CAD build for the part. Positions are in the model's coordinates, mm. Give positions to 0.01 mm unless a question says otherwise; leave off trailing zeros. Write each loop counter-clockwise with the first axis right and the second up, starting at its lowest first coordinate (ties: lowest second). Pieces come first, ordered by that corner, then holes. Notation, with made-up numbers: (-26.5, 51.5) - (-8.5, 51.5) arc R10 cw to (-8.5, 55.5) - close; hole circle Ø8 at (43, -17.5). An arc over 180 degrees is marked (long way). Put each result on its own line as item: value. Start each with the question number.
1. Wall check: line 1 (Y direction, x = 37, z = -8); line 2 (Z direction, x = 22.5, y = 0.25); line 3 (Z direction, x = -34, y = 0.8). Give the ranges that are in metal, low to high.
2. Cut at B-B on x = -23. List the corners of the cut face in (y, z), and give its area (3 significant figures).
3. Cut at A-A on z = 21.5. List the corners of the cut face in (x, y).
4. Drop a flat-ended pin along its axis: pin 1 (3 mm diameter, centred on x = 3, z = -3, fed in from +Y). Give the stop position or say it passes through.
from build123d import *

# Parameters (mm, degrees)
SKETCH1_W           = 81
SKETCH1_H           = 50.5
BOSS_EXTRUDE1_DEPTH = 2
SKETCH2_W           = 50.5
SKETCH2_H           = 1
EXTRUDE_THIN1_DEPTH = 1
FILLET4_START       = -26
FILLET4_DEPTH       = 52
FILLET4_START_2     = -25.25
FILLET4_2_DEPTH     = 50.5
FILLET8_R           = 6
BOSS_EXTRUDE2_DEPTH = 0.5


with BuildPart() as part:
    # Sketch1 → Boss-Extrude1 (new body)
    with BuildSketch(Plane(origin=(0, 0, 0), x_dir=(1, 0, 0), z_dir=(0, 1, 0))):
        Rectangle(SKETCH1_W, SKETCH1_H)
    extrude(amount=BOSS_EXTRUDE1_DEPTH)

    # Sketch2 → Extrude-Thin1 (add)
    with BuildSketch(Plane(origin=(40.5, 0, 0), x_dir=(0, 0, -1), z_dir=(1, 0, 0))):
        with Locations((0, 1)):
            Rectangle(SKETCH2_W, SKETCH2_H)
    extrude_thin1 = extrude(amount=EXTRUDE_THIN1_DEPTH)

    # Mirror1: Extrude-Thin1 across plane
    add(extrude_thin1.mirror(Plane(origin=(0, 0, 0), x_dir=(0, 0, 1), z_dir=(1, 0, 0))))

    # Fillet4: read off the stored shape, not the designer's step
    # Fillet4 outline → Fillet4 (cut)
    with BuildSketch(Plane.XY.offset(FILLET4_START)):
        with BuildLine():
            Line((-41.5, 0.5), (-41, 0.5))
            ThreePointArc((-41, 0.5), (-41.353553391, 0.646446609), (-41.5, 1))
            Line((-41.5, 1), (-41.5, 0.5))
        make_face()
        with BuildLine():
            Line((-41.5, 1.5), (-41.5, 1))
            ThreePointArc((-41.5, 1), (-41.353553391, 1.353553391), (-41, 1.5))
            Line((-41, 1.5), (-41.5, 1.5))
        make_face()
        with BuildLine():
            Line((41.5, 1.5), (41, 1.5))
            ThreePointArc((41, 1.5), (41.353553391, 1.353553391), (41.5, 1))
            Line((41.5, 1), (41.5, 1.5))
        make_face()
        with BuildLine():
            Line((41.5, 0.5), (41.5, 1))
            ThreePointArc((41.5, 1), (41.353553391, 0.646446609), (41, 0.5))
            Line((41, 0.5), (41.5, 0.5))
        make_face()
    extrude(amount=FILLET4_DEPTH, mode=Mode.SUBTRACT)

    # Fillet4 2 outline → Fillet4 2 (add)
    with BuildSketch(Plane.XY.offset(FILLET4_START_2)):
        with BuildLine():
            Line((-40.5, 0.5), (-41, 0.5))
            ThreePointArc((-41, 0.5), (-40.646446609, 0.353553391), (-40.5, 0))
            Line((-40.5, 0), (-40.5, 0.5))
        make_face()
        with BuildLine():
            ThreePointArc((-40.5, 2), (-40.646446609, 1.646446609), (-41, 1.5))
            Line((-41, 1.5), (-40.5, 1.5))
            Line((-40.5, 1.5), (-40.5, 2))
        make_face()
        with BuildLine():
            Line((40.5, 1.5), (41, 1.5))
            ThreePointArc((41, 1.5), (40.646446609, 1.646446609), (40.5, 2))
            Line((40.5, 2), (40.5, 1.5))
        make_face()
        with BuildLine():
            ThreePointArc((40.5, 0), (40.646446609, 0.353553391), (41, 0.5))
            Line((41, 0.5), (40.5, 0.5))
            Line((40.5, 0.5), (40.5, 0))
        make_face()
    extrude(amount=FILLET4_2_DEPTH)

    # Fillet8
    # the kernel refuses this fillet: 6 mm, written as the material it takes off along each edge
    with BuildSketch(Plane(origin=(-51.680339887, 2, -25.25), x_dir=(0, -1, 0), z_dir=(1, 0, 0))) as fillet8_piece_1:
        with BuildLine():
            CenterArc((6, -4.472135955), FILLET8_R, 131.810314896, 48.189685104)
            Line((0, -4.472135955), (-0.12, -4.472135955))
            Line((-0.12, -4.472135955), (-0.12, 0))
            Line((-0.12, 0), (0, 0.12))
            ThreePointArc((0, 0.12), (1, 0.12), (1.92, 0.089442719))
            Line((1.92, 0.089442719), (2, 0))
        make_face()
    extrude(amount=103.360679775, mode=Mode.SUBTRACT)

    # Sketch3 → Boss-Extrude2 (add)
    with BuildSketch(Plane(origin=(0, 2, 0), x_dir=(1, 0, 0), z_dir=(0, 1, 0))):
        Polygon((0, 20.777864045), (-0.527934032, 20.249930013), (0.527934032, 20.249930013), align=None)
        Polygon((-4.470357419, 16.307506626), (4.470357419, 16.307506626), (3.779119733, 16.998744312), (-3.779119733, 16.998744312), align=None)
        Polygon((-1.175607402, 19.602256643), (1.175607402, 19.602256643), (1.863999283, 18.913864762), (-1.863999283, 18.913864762), align=None)
        Polygon((-2.621779089, 18.156084956), (2.621779089, 18.156084956), (3.215777687, 17.562086358), (-3.215777687, 17.562086358), align=None)
    extrude(amount=BOSS_EXTRUDE2_DEPTH)


solid = part.part
Report:
1. line 1: y = 0 to 2
1. line 2: z = -25.01 to 25.25
1. line 3: z = -24.38 to 25.25
2. outline: (0, -25.25) arc R6 ccw to (2, -20.78) - (2, 25.25) - (0, 25.25) - close
2. area: 98.3 mm²
3. outline: (-41, 0.5) arc R0.5 cw to (-40.5, 0) - (40.5, 0) arc R0.5 cw to (41, 0.5) arc R0.5 ccw to (41, 1.5) arc R0.5 cw to (40.5, 2) - (-40.5, 2) arc R0.5 cw to (-41, 1.5) arc R0.5 ccw to start
4. pin 1: stops at y = 2
